Could you check a few things on this drawing? It's one solid part, dimensions in mm from its lowest x, y, z. A direction names the side the tool comes from. Round coordinates to 2 decimals unless told otherwise and drop trailing zeros. Loops run counter-clockwise (first coordinate to the right, second up) from the corner with the lowest first, then second, coordinate; pieces in that order, holes last. Notation, with made-up numbers: M 52.25,50 L 94.25,50 A27 ccw 94.25,80 Z; hole C 87.25,60 d2. An arc over 180 degrees is marked long. Return JSON: item names as keys, results as strings.
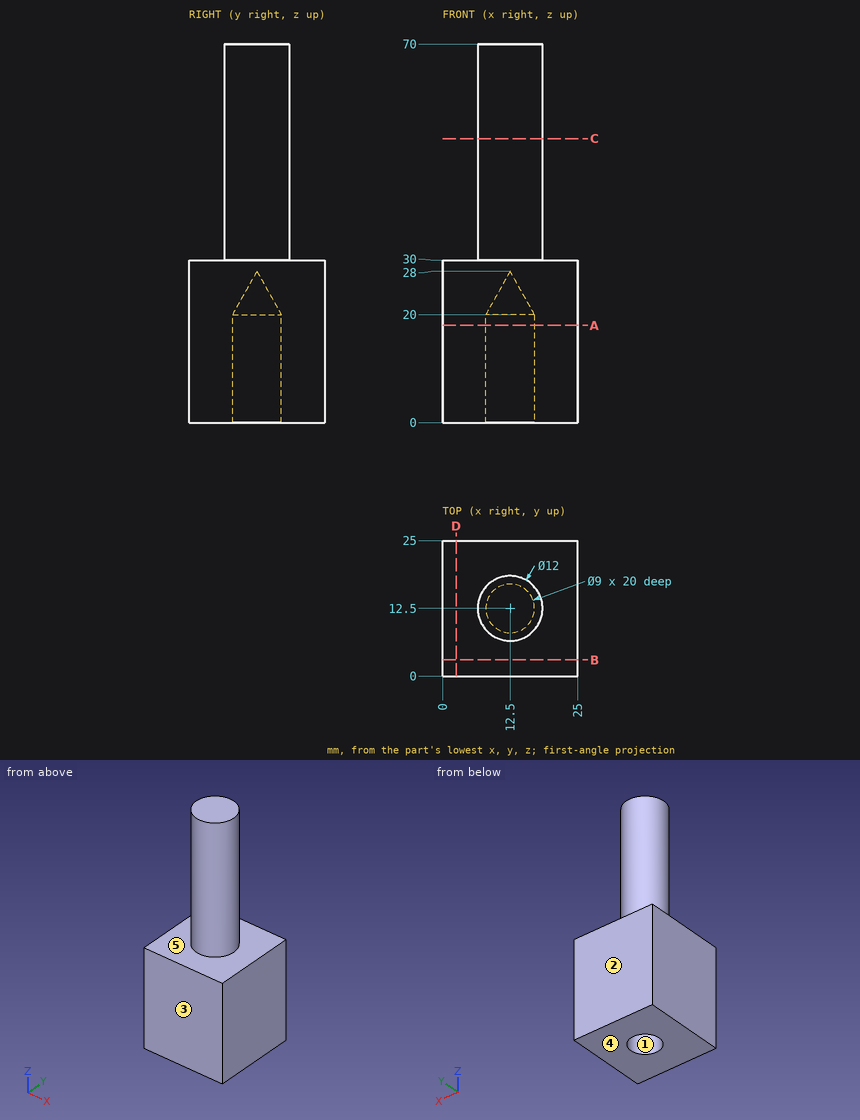
Q1. I'm going to push flat-ended pins straight in: pin 1 Ø4 at (x, y) = (3.5, 17.5) entering from +Z; pin 2 Ø5.5 at (x, y) = (12.5, 12.5) entering from -Z. Where does each tip first touch, or does it pass through?
Results:
{"pin 1": "stops at z = 30", "pin 2": "stops at z = 23.11"}
Q2. On a 3-axis mill with a long thin cutter (end or side, diameter ignored), from which of +Z, -Z, +X, -X, +Y, -Y can I reach the whole of each face in a straight line? I mean the marked faces 4 and 5. Say none if no direction works.
Results:
{"face 4": "-Z, +X, -X, +Y, -Y", "face 5": "+Z"}
Q3. Suppose I cut it at B-B, the plane y = 3. Please give me the cut outline in (x, z), plus the area to 3 significant figures.
Results:
{"outline": "M 0,0 L 25,0 L 25,30 L 0,30 Z", "area": "750 mm2"}
Q4. Suppose I cut it at A-A, the plane z = 18. Please give me the cut outline in (x, y), plus the area to 3 significant figures.
Results:
{"outline": "M 0,0 L 25,0 L 25,25 L 0,25 Z; hole C 12.5,12.5 d9", "area": "561 mm2"}
Q5. Suppose I cut it at C-C, the plane z = 52.5. Please give me the cut outline in (x, y), plus the area to 3 significant figures.
Results:
{"outline": "C 12.5,12.5 d12", "area": "113 mm2"}
Q6. Thinking about a two-plate mould opening in Y: for the marked faces 1, 2 and 3, which applies, pulls with the +Y half, pulls with the -Y half, needs draft (parallel to the pull), parting line crosses it, or undercut?
Results:
{"face 1": "undercut", "face 2": "pulls with the +Y half", "face 3": "pulls with the -Y half"}
Q7. If I drill on line 1 along Y through (x, z) = (12.5, 15.75); line 2 along Z through (x, y) = (10, 21.75), over which ranges is the centre line in solid material (lowest first)?
Results:
{"line 1": "y = 0 to 8, 17 to 25", "line 2": "z = 0 to 30"}
